from build123d import *

# Parameters (mm, degrees)
SKETCH1_R                   = 6.35
EXTRUDE1_DEPTH              = 56.35625
F_1_4_20_TAPPED_HOLE1_D     = 5.1054
F_1_4_20_TAPPED_HOLE1_DEPTH = 19.05
F_1_4_20_TAPPED_HOLE1_TIP   = 1.533816902
F_1_4_20_TAPPED_HOLE2_D     = 5.1054
F_1_4_20_TAPPED_HOLE2_DEPTH = 19.05
F_1_4_20_TAPPED_HOLE2_TIP   = 1.533816902


with BuildPart() as part:
    # Sketch1 → Extrude1 (new body, symmetric)
    with BuildSketch(Plane.XY):
        Circle(SKETCH1_R)
    extrude(amount=EXTRUDE1_DEPTH, both=True)

    # 1/4-20 Tapped Hole1
    with Locations(Plane.XY.offset(56.35625)):
        with Locations((0, 0)):
            Hole(F_1_4_20_TAPPED_HOLE1_D / 2, depth=F_1_4_20_TAPPED_HOLE1_DEPTH)
            with Locations((0, 0, -(F_1_4_20_TAPPED_HOLE1_DEPTH + F_1_4_20_TAPPED_HOLE1_TIP / 2))):  # 118° drill point
                Cone(0, F_1_4_20_TAPPED_HOLE1_D / 2, F_1_4_20_TAPPED_HOLE1_TIP, mode=Mode.SUBTRACT)

    # 1/4-20 Tapped Hole2
    with Locations(Plane(origin=(0, 0, -56.35625), x_dir=(-1, 0, 0), z_dir=(0, 0, -1))):
        with Locations((0, 0)):
            Hole(F_1_4_20_TAPPED_HOLE2_D / 2, depth=F_1_4_20_TAPPED_HOLE2_DEPTH)
            with Locations((0, 0, -(F_1_4_20_TAPPED_HOLE2_DEPTH + F_1_4_20_TAPPED_HOLE2_TIP / 2))):  # 118° drill point
                Cone(0, F_1_4_20_TAPPED_HOLE2_D / 2, F_1_4_20_TAPPED_HOLE2_TIP, mode=Mode.SUBTRACT)


solid = part.part
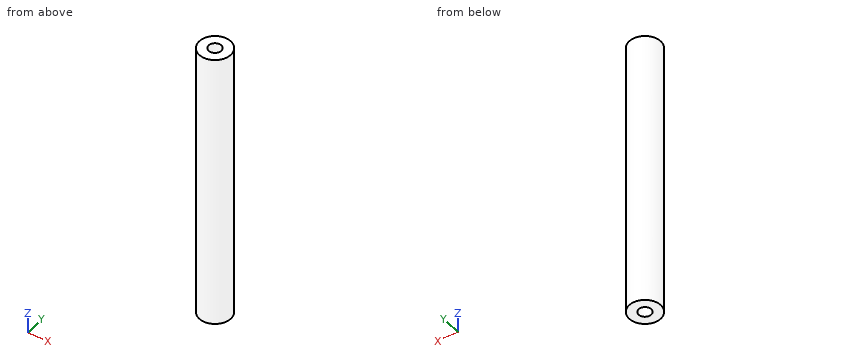
Geometry: final body of the model. Coordinates: model frame, mm. Round coordinates to 2 decimals unless told otherwise and drop trailing zeros. Order: outer loops, then holes, each group sorted by start corner. A loop starts at its lowest first (then second) coordinate and runs counter-clockwise, first axis right, second up. Notation, with made-up numbers: (48.25, 73.5) - (72.25, 73.5) arc R21 cw to (72.25, 100.5) - close; hole circle Ø7 at (18, -6). An arc over 180 degrees is marked (long way). Write each question's results on one line, items separated by ' | '.
Item 1: Material intervals for line 1 along Y through (x, z) = (0, 46.5); line 2 along Y through (x, z) = (-2, 43.5); line 3 along X through (y, z) = (-0.25, -6), sorted ascending. Write a range as [from, to].
Completed:
line 1: [-6.35, -2.55], [2.55, 6.35] | line 2: [-6.03, -1.59], [1.59, 6.03] | line 3: [-6.35, 6.35]
Item 2: Section A-A, the plane z = 10.5. Return the cut outline in (x, y), and give its area (3 significant figures).
Completed:
outline: circle Ø12.7 at (0, 0) | area: 127 mm^2
Item 3: First-contact query: pin 1 Ø4 at (y, z) = (3.5, -43.5) entering from -X; pin 2 Ø2 at (x, z) = (-4, 21) entering from +Y; pin 3 Ø3 at (x, z) = (-3.5, 19) entering from -Y. Flat tips, straight axial feed; report the tip coordinate or a pass-through.
Completed:
pin 1: x = -6.17 | pin 2: y = 5.6 | pin 3: y = -6.03
Item 4: Section B-B, the plane x = 3.75. Return the cut outline in (y, z).
Completed:
outline: (-5.12, -56.36) - (5.12, -56.36) - (5.12, 56.36) - (-5.12, 56.36) - close
